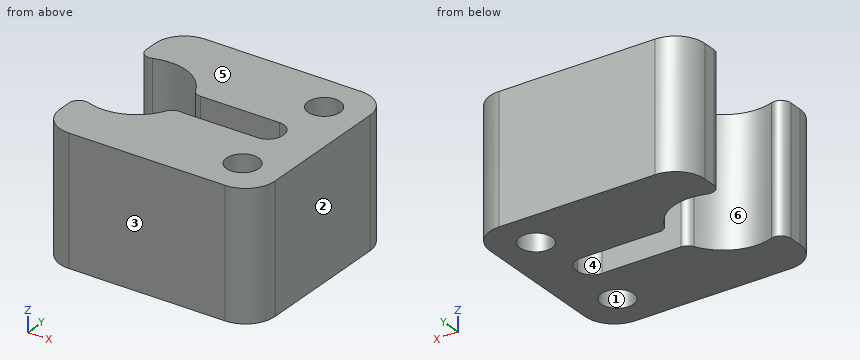
```python
from build123d import *

# Parameters (mm, degrees)
ESQUISSE1_W                  = 22
ESQUISSE1_H                  = 20
BOSS_EXTRU_1_DEPTH           = 13
ESQUISSE2_R                  = 1.65
ENL_V_MAT_EXTRU_1_DEPTH      = 1
ENL_V_MAT_EXTRU_1_DEPTH_BACK = 14
ESQUISSE4_W                  = 12
ESQUISSE4_H                  = 3.2
ENL_V_MAT_EXTRU_2_DEPTH      = 13
CONG_1_R                     = 1
CONG_2_R                     = 3
CONG_3_R                     = 1.5


with BuildPart() as part:
    # Esquisse1 → Boss.-Extru.1 (new body)
    with BuildSketch(Plane.XY):
        with Locations((11, 10)):
            Rectangle(ESQUISSE1_W, ESQUISSE1_H)
    extrude(amount=BOSS_EXTRU_1_DEPTH)

    # Esquisse2 → Enlèv. mat.-Extru.1 (cut, two sides)
    with BuildSketch(Plane.XY.offset(13)) as enl_v_mat_extru_1_sk:
        with Locations((18, 16)):
            Circle(ESQUISSE2_R)
        with Locations((18, 4)):
            Circle(ESQUISSE2_R)
        with BuildLine():
            Line((0, 6), (0, 14))
            ThreePointArc((0, 14), (8, 10), (0, 6))
        make_face()
    extrude(amount=ENL_V_MAT_EXTRU_1_DEPTH, mode=Mode.SUBTRACT)
    extrude(enl_v_mat_extru_1_sk.sketch, amount=-ENL_V_MAT_EXTRU_1_DEPTH_BACK, mode=Mode.SUBTRACT)

    # Esquisse4 → Enlèv. mat.-Extru.2 (cut)
    with BuildSketch(Plane.XY.offset(13)):
        with Locations((12, 10)):
            Rectangle(ESQUISSE4_W, ESQUISSE4_H)
    extrude(amount=-ENL_V_MAT_EXTRU_2_DEPTH, mode=Mode.SUBTRACT)

    # Congé1
    cong_1_edges = [part.edges().sort_by_distance(p)[0] for p in [
        (0, 14, 6.5),
        (0, 6, 6.5),
        (7.737087713, 11.6, 6.5),
        (7.737087713, 8.4, 6.5),
    ]]
    fillet(cong_1_edges, radius=CONG_1_R)

    # Congé2
    cong_2_edges = [part.edges().sort_by_distance(p)[0] for p in [
        (0, 20, 6.5),
        (22, 20, 6.5),
        (22, 0, 6.5),
        (0, 0, 6.5),
    ]]
    fillet(cong_2_edges, radius=CONG_2_R)

    # Congé3
    cong_3_edges = [part.edges().sort_by_distance(p)[0] for p in [
        (18, 8.4, 6.5),
        (18, 11.6, 6.5),
    ]]
    fillet(cong_3_edges, radius=CONG_3_R)


solid = part.part
```
CAD build for the part. Positions are in the model's coordinates, mm. Face numbers are marked on the shaded views. A direction names the side the tool comes from. Coordinates: 2 decimals unless noted, no trailing zeros. Order: outer loops, then holes, each group sorted by start corner. A loop starts at its lowest first (then second) coordinate and runs counter-clockwise, first axis right, second up. Notation, with made-up numbers: M 81,22 L 124,22 A25 ccw 124,49 Z; hole C -0.75,25.5 d7. An arc over 180 degrees is marked long. Answer as CSV lines item,"result".
1) Cut at D-D (y = 6). List the corners of the cut face in (x, z), then the cut area to 3 significant figures.
Verdict:
outline,"M 6,0 L 22,0 L 22,13 L 6,13 Z"
area,"208 mm2"
2) Cut at A-A (y = 16). List the corners of the cut face in (x, z).
Verdict:
outline,"M 0,0 L 16.35,0 L 16.35,13 L 0,13 Z; M 19.65,0 L 22,0 L 22,13 L 19.65,13 Z"
3) 3-axis set-ups, long thin cutter, end or side, ignore diameter. For the marked faces 4, 5 and 6: which of +Z, -Z, +X, -X, +Y, -Y reach the whole face in a straight line?
Verdict:
face 4,"+Z, -Z, -X"
face 5,"+Z, +X, -X, +Y, -Y"
face 6,"+Z, -Z"
4) Cut at C-C (z = 2). List the corners of the cut face in (x, y).
Verdict:
outline,"M 0,3 A3 ccw 3,0 L 19,0 A3 ccw 22,3 L 22,17 A3 ccw 19,20 L 3,20 A3 ccw 0,17 L 0,15.66 A1 ccw 1.33,14.71 A5 cw 7.51,12.17 A1 ccw 8.41,11.6 L 16.5,11.6 A1.5 cw 18,10.1 L 18,9.9 A1.5 cw 16.5,8.4 L 8.41,8.4 A1 ccw 7.51,7.83 A5 cw 1.33,5.29 A1 ccw 0,4.34 Z; hole C 18,4 d3.3; hole C 18,16 d3.3"
5) Mould opens along X. For the marked faces 1, 2 and 3 say: released by +X, released by -X, zero draft, split by the parting line, or undercut.
Verdict:
face 1,"undercut"
face 2,"released by +X"
face 3,"zero draft"
6) Drill centre lines: L1, parallel to Y at x = 16, z = 9.25; L2, parallel to Y at x = 3, z = 10; L3, parallel to Y at x = 18.5, z = 10.25. Where is each one in solid material? Low to high. Write a range as from..to.
Verdict:
L1,"0..8.4, 11.6..20"
L2,"0..5, 15..20"
L3,"0..2.43, 5.57..14.43, 17.57..20"
7) Cut at B-B (x = 6.5). List the corners of the cut face in (y, z), then the cut area to 3 significant figures.
Verdict:
outline,"M 0,0 L 6.43,0 L 6.43,13 L 0,13 Z; M 13.57,0 L 20,0 L 20,13 L 13.57,13 Z"
area,"167 mm2"
